CAD build for the part. Positions are in the model's coordinates, mm. A direction names the side the tool comes from. Round coordinates to 2 decimals unless told otherwise and drop trailing zeros. Order: outer loops, then holes, each group sorted by start corner. A loop starts at its lowest first (then second) coordinate and runs counter-clockwise, first axis right, second up. Notation, with made-up numbers: M 12.5,-5 L 60.5,-5 A26 cw 60.5,34 Z; hole C 56,-3.5 d2. An arc over 180 degrees is marked long. Answer as a JSON object with one key per item and string values. Group by question number.
```python
from build123d import *

# Parameters (mm, degrees)
F0_W     = 98.4
F0_H     = 108.4
F1_DEPTH = 1.2
F0_W_2   = 100
F0_H_2   = 110
F2_DEPTH = 100
F3_R     = 2.2
F4_R     = 3


with BuildPart() as f1:
    # F0 (on Top) → F1 (new body)
    with BuildSketch(Plane.XY):
        Rectangle(F0_W, F0_H)
    extrude(amount=F1_DEPTH)

    # F0 (on Top) → F2 (join)
    with BuildSketch(Plane.XY):
        Rectangle(F0_W_2, F0_H_2)
        Rectangle(F0_W, F0_H, mode=Mode.SUBTRACT)
    extrude(amount=F2_DEPTH)

    # F3
    f3_edges = [f1.edges().sort_by_distance(p)[0] for p in [
        (49.2, 0, 1.2),
        (0, 54.2, 1.2),
        (-49.2, 0, 1.2),
        (0, -54.2, 1.2),
        (-49.2, 54.2, 50.6),
        (-49.2, -54.2, 50.6),
        (49.2, -54.2, 50.6),
        (49.2, 54.2, 50.6),
    ]]
    fillet(f3_edges, radius=F3_R)

    # F4
    f4_edges = [f1.edges().sort_by_distance(p)[0] for p in [
        (50, 55, 50),
        (50, 0, 0),
        (0, 55, 0),
        (-50, 0, 0),
        (0, -55, 0),
        (-50, 55, 50),
        (-50, -55, 50),
        (50, -55, 50),
    ]]
    fillet(f4_edges, radius=F4_R)


solid = f1.part
```
Item 1: Two-plate mould, pull along X, no slides. Class faces 3 (the face through (-49.2, -1, 51)), 4 (the face through (0.66, -54.14, 0.9)), 5 (the face through (-50, -1, 51)): +X half, -X half, draft (parallel to the pull), parting line (faces both ways), or undercut.
Item 2: Drill centre lines: line 1 (X direction, y = 5.5, z = 65); line 2 (Y direction, x = 27, z = 20.5); line 3 (Z direction, x = 25, y = 22.5). Where is each one in solid material? Low to high. Write a range as [from, to].
Item 3: Cut at C-C, the plane y = -14.5. Give the cut face in (x, z).
Item 4: Cut at B-B, the plane x = -43.5. Give the cut face in (y, z).
Item 5: Cut at A-A, the plane z = 47. Give the cut face in (x, y), and give its area (3 significant figures).
Item 6: 3-axis set-ups, long thin cutter, end or side, ignore diameter. For faces 1 (the face through (49.14, 0.73, 0.9)), 2 (the face through (-1, 54.2, 51)): which of +Z, -Z, +X, -X, +Y, -Y reach the whole face in a straight line?
Item 7: Flat gauge pin, fed straight in: pin 1 Ø5 at (x, y) = (25, 33) entering from +Z. Where does the tip first touch, or does it go through?
Response values:
{
 "1": {"face 3": "undercut", "face 4": "draft", "face 5": "-X half"},
 "2": {"line 1": "[-50, -49.2], [49.2, 50]", "line 2": "[-55, -54.2], [54.2, 55]", "line 3": "[0, 1.2]"},
 "3": {"outline": "M -50,3 A3 ccw -47,0 L 47,0 A3 ccw 50,3 L 50,100 L 49.2,100 L 49.2,3.4 A2.2 cw 47,1.2 L -47,1.2 A2.2 cw -49.2,3.4 L -49.2,100 L -50,100 Z"},
 "4": {"outline": "M -55,3 A3 ccw -52,0 L 52,0 A3 ccw 55,3 L 55,100 L 54.2,100 L 54.2,3.4 A2.2 cw 52,1.2 L -52,1.2 A2.2 cw -54.2,3.4 L -54.2,100 L -55,100 Z"},
 "5": {"outline": "M -50,-52 A3 ccw -47,-55 L 47,-55 A3 ccw 50,-52 L 50,52 A3 ccw 47,55 L -47,55 A3 ccw -50,52 Z; hole M -49.2,-52 A2.2 ccw -47,-54.2 L 47,-54.2 A2.2 ccw 49.2,-52 L 49.2,52 A2.2 ccw 47,54.2 L -47,54.2 A2.2 ccw -49.2,52 Z", "area": "330 mm^2"},
 "6": {"face 1": "-Z, +X, +Y, -Y", "face 2": "+Z"},
 "7": {"pin 1": "z = 1.2"}
}
